Geometry: final body of the model. Coordinates: model frame, mm. Face numbers are marked on the shaded views. A direction names the side the tool comes from. Give positions to 0.01 mm unless a question says otherwise; leave off trailing zeros. Order: outer loops, then holes, each group sorted by start corner. A loop starts at its lowest first (then second) coordinate and runs counter-clockwise, first axis right, second up. Notation, with made-up numbers: (47, 38) - (77, 38) arc R27 ccw to (77, 67) - close; hole circle Ø11 at (-18, 35). An arc over 180 degrees is marked (long way). Put each result on its own line as item: value. Start each with the question number.
1. Ray query, line 1 along X through (y, z) = (-47.5, 30.5); line 2 along X through (y, z) = (-52.5, 227); line 3 along Z through (x, y) = (57, -21). Return the intervals inside material, ascending. Write a range as from..to.
2. Section B-B on z = 195.5. Return the cut outline in (x, y), plus the area to 3 significant figures.
3. Section D-D on x = 108. Return the cut outline in (y, z).
4. First-contact query: P1, Ø8, axis at y = -34.5, z = 3.5, coming from the +X side; P2, Ø8, axis at y = -62.5, z = 3.5, coming from the -X side; P3, Ø5, axis at x = 73, y = -96.5, coming from the +Z side. Flat tips, straight axial feed; report the tip coordinate or a pass-through.
5. Section A-A on z = 53. Return the cut outline in (x, y), plus the area to 3 significant figures.
6. Section C-C on y = -29.5. Return the cut outline in (x, z).
7. Mould query, pull axis X, two halves, no side actions, for the marked faces 1, 2 and 3. Classes: pulls with the +X half, pulls with the -X half, needs draft (parallel to the pull), parting line crosses it, or undercut.
8. Set-up query: the marked faces 4 and 5. Return all of +Z, -Z, +X, -X, +Y, -Y with unobstructed straight access to the full face (end or side cutting, diameter ignored); none if empty.
from build123d import *

# Parameters (mm, degrees)
F1_DEPTH = 130


with BuildPart() as f1:
    # F0 (on Front) → F1 (new body)
    with BuildSketch(Plane.XZ):
        with BuildLine():
            Line((0, 10), (0, 0))
            Line((0, 0), (15.757065, 0))
            Line((15.757065, 0), (15.757065, 205.330478))
            ThreePointArc((15.757065, 205.330478), (12.938265, 207.591795), (10.243875, 210))
            Line((10.243875, 210), (10.243875, 10))
            Line((10.243875, 10), (0, 10))
        make_face()
        with BuildLine():
            ThreePointArc((10.243875, 210), (12.938265, 207.591795), (15.757065, 205.330478))
            ThreePointArc((15.757065, 205.330478), (56.464246, 191.519328), (97.300157, 204.94508))
            ThreePointArc((97.300157, 204.94508), (100.728563, 207.674159), (103.973635, 210.618874))
            ThreePointArc((103.973635, 210.618874), (119.250429, 232.892095), (124.626733, 259.36042))
            Line((124.626733, 259.36042), (116.784884, 259.36042))
            ThreePointArc((116.784884, 259.36042), (113.592055, 240.048628), (104.353374, 222.792145))
            ThreePointArc((104.353374, 222.792145), (56.784884, 199.36042), (9.216394, 222.792145))
            ThreePointArc((9.216394, 222.792145), (-0.022288, 240.048628), (-3.215116, 259.36042))
            Line((-3.215116, 259.36042), (-11.056966, 259.36042))
            ThreePointArc((-11.056966, 259.36042), (-5.50454, 232.480237), (10.243875, 210))
        make_face()
        with BuildLine():
            ThreePointArc((103.973635, 210.618874), (100.728563, 207.674159), (97.300157, 204.94508))
            Line((97.300157, 204.94508), (97.300157, 0))
            Line((97.300157, 0), (113.569767, 0.618874))
            Line((113.569767, 0.618874), (113.569767, 10.618874))
            Line((113.569767, 10.618874), (103.973635, 10.618874))
            Line((103.973635, 10.618874), (103.973635, 210.618874))
        make_face()
    extrude(amount=F1_DEPTH)


solid = f1.part
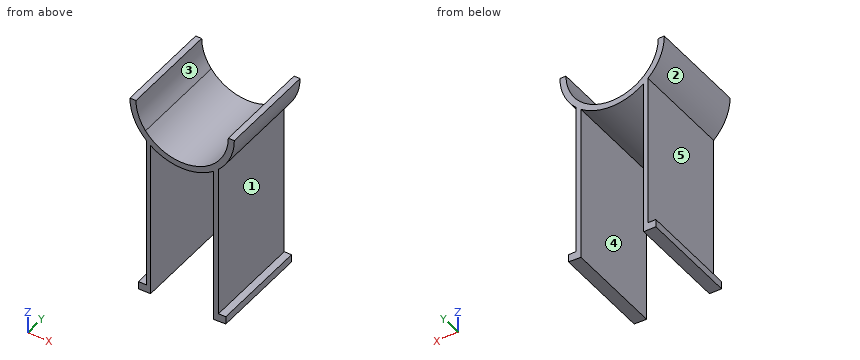
Resolved:
1. line 1: 10.24..15.76, 97.3..103.97
1. line 2: -2.84..6.26, 107.31..116.41
1. line 3: 191.52..199.36
2. outline: (10.24, -130) - (15.76, -130) - (15.76, 0) - (10.24, 0) - close; (33.89, -130) - (79.68, -130) - (79.68, 0) - (33.89, 0) - close; (97.3, -130) - (103.97, -130) - (103.97, 0) - (97.3, 0) - close
2. area: 7,540 mm^2
3. outline: (-130, 0.41) - (0, 0.41) - (0, 10.62) - (-130, 10.62) - close; (-130, 214.87) - (0, 214.87) - (0, 228.1) - (-130, 228.1) - close
4. P1: x = 113.57
4. P2: x = 0
4. P3: z = 202.35
5. outline: (10.24, -130) - (15.76, -130) - (15.76, 0) - (10.24, 0) - close; (97.3, -130) - (103.97, -130) - (103.97, 0) - (97.3, 0) - close
5. area: 1,580 mm^2
6. outline: (-11.06, 259.36) arc R67.84 ccw to (10.24, 210) - (10.24, 10) - (0, 10) - (0, 0) - (15.76, 0) - (15.76, 205.33) arc R67.84 ccw to (97.3, 204.95) - (97.3, 0) - (113.57, 0.62) - (113.57, 10.62) - (103.97, 10.62) - (103.97, 210.62) arc R67.84 ccw to (124.63, 259.36) - (116.78, 259.36) arc R60 cw to (9.22, 222.79) arc R60 cw to (-3.22, 259.36) - close
7. face 1: pulls with the +X half
7. face 2: pulls with the -X half
7. face 3: undercut
8. face 4: -Z, +Y, -Y
8. face 5: -X, +Y, -Y
